Part print with two shaded views. Sizes in mm from the minimum x, y, z corner. A direction names the side the tool comes from. Coordinates: 2 decimals unless noted, no trailing zeros. Write each loop counter-clockwise with the first axis right and the second up, starting at its lowest first coordinate (ties: lowest second). Pieces come first, ordered by that corner, then holes. Notation, with made-up numbers: (-25, 26.5) - (-6, 26.5) arc R26 cw to (-6, 41.5) - close; hole circle Ø10 at (7.5, 4.5). An arc over 180 degrees is marked (long way). One line per question, with ' | ' between items. Start each with the question number.
1. Which spindle directions (+Z, -Z, +X, -X, +Y, -Y) get a long thin tool onto all of the face, cutting with end or side? Do the marked faces 4, 5 and 6. Say none if no direction does.
2. Band-saw the part on A-A, the plane y = 3.75. Write the cut outline in (x, z), then the cut area to 3 significant figures.
3. Two-plate mould, pull along Z, no slides. Class the marked faces 1, 2 and 3: +Z half, -Z half, draft (parallel to the pull), parting line (faces both ways), or undercut.
4. Band-saw the part on C-C, the plane z = 25. Write the cut outline in (x, y).
5. Band-saw the part on B-B, the plane x = 30.5. Give the number of separate pieces and of enclosed holes in the cut face.
6. Band-saw the part on D-D, the plane x = 16.5. Write the cut outline in (y, z).
7. Flat gauge pins, fed straight in: P1, Ø2, axis at y = 6, z = 6, coming from the -X side; P2, Ø4.5, axis at x = 17, y = 5, coming from the -Z side; P3, Ø8, axis at x = 16.5, z = 11.02, coming from the -Y side. Where does each tip first touch, or does it go through?
8. Probe line 1 (X direction, y = 6.75, z = 13.25) (1 decimal); line 2 (X direction, y = 1.75, z = 15.75) (1 decimal); line 3 (Z direction, x = 23.5, y = 2.75). List the from-to ranges inside material, lowest first.
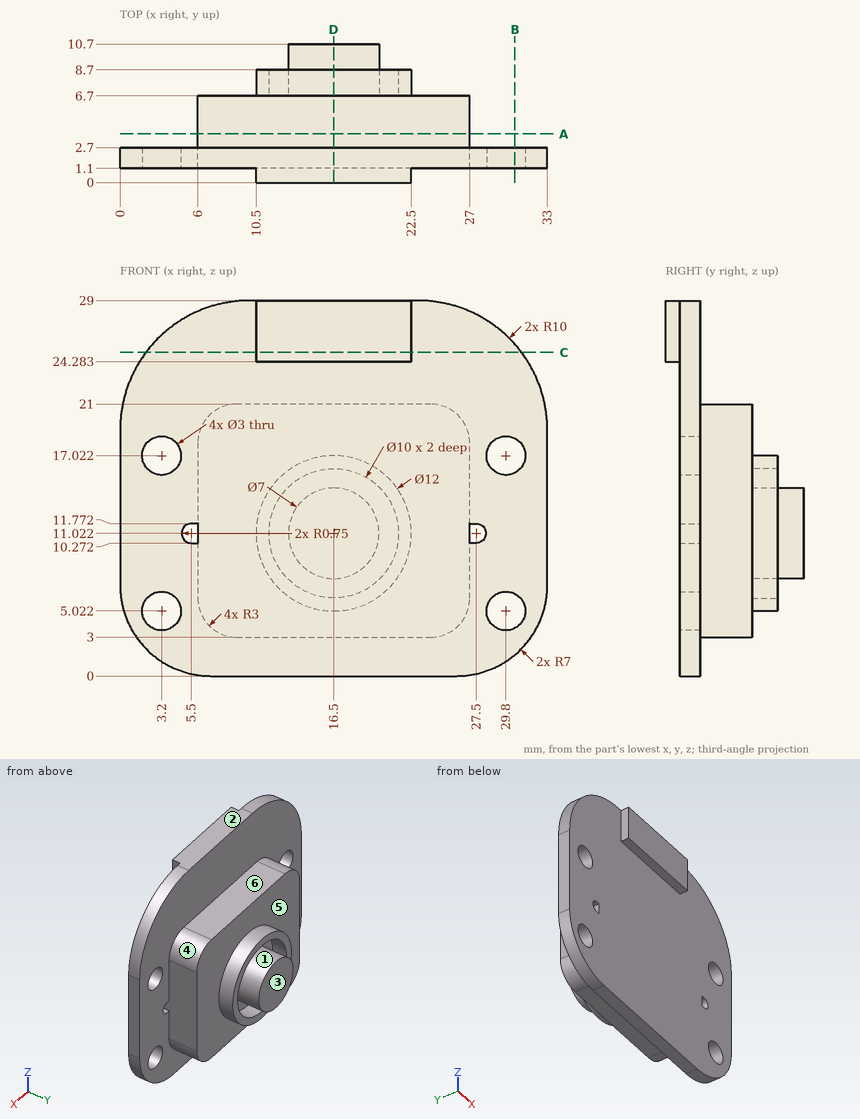
Filled in:
1) face 4: +Z, +X, +Y | face 5: +Y | face 6: +Z, +X, -X, +Y
2) outline: (6, 6) arc R3 ccw to (9, 3) - (24, 3) arc R3 ccw to (27, 6) - (27, 18) arc R3 ccw to (24, 21) - (9, 21) arc R3 ccw to (6, 18) - close | area: 370 mm²
3) face 1: undercut | face 2: +Z half | face 3: draft
4) outline: (2, 1.1) - (10.5, 1.1) - (10.5, 0) - (22.5, 0) - (22.5, 1.1) - (31, 1.1) - (31, 2.7) - (2, 2.7) - close
5) separate pieces: 3 | enclosed holes: 0
6) outline: (0, 24.28) - (1.1, 24.28) - (1.1, 0) - (2.7, 0) - (2.7, 3) - (6.7, 3) - (6.7, 5.02) - (8.7, 5.02) - (8.7, 6.02) - (6.7, 6.02) - (6.7, 7.52) - (10.7, 7.52) - (10.7, 14.52) - (6.7, 14.52) - (6.7, 16.02) - (8.7, 16.02) - (8.7, 17.02) - (6.7, 17.02) - (6.7, 21) - (2.7, 21) - (2.7, 29) - (0, 29) - close
7) P1: stops at x = 6 | P2: stops at z = 3 | P3: stops at y = 1.1
8) line 1: x = 10.9 to 12, 13.8 to 19.2, 21 to 22.1 | line 2: x = 0 to 2.4, 4 to 29, 30.6 to 33 | line 3: z = 3 to 21
